Build history of the part. All positions in model axes, mm. Face numbers are marked on the shaded views. A direction names the side the tool comes from. Give positions to 0.01 mm unless a question says otherwise; leave off trailing zeros. Write each loop counter-clockwise with the first axis right and the second up, starting at its lowest first coordinate (ties: lowest second). Pieces come first, ordered by that corner, then holes. Notation, with made-up numbers: (32.5, -9) -> (39.5, -9) arc R16 cw to (39.5, 14) -> close; hole circle Ø8 at (-39, 61). An arc over 180 degrees is marked (long way). Put each result on its own line as item: value.
Autodesk Inventor part; units mm, degrees
ref_plane "YZ Plane" through (0, 0, 0) normal (1, 0, 0) x (0, 1, 0)
ref_plane "XZ Plane" through (0, 0, 0) normal (0, 1, 0) x (-1, 0, 0)
ref_plane "XY Plane" through (0, 0, 0) normal (0, 0, 1) x (1, 0, 0)
sketch "Sketch1" plane through (0, 0, 0) normal (0, 0, 1) x (1, 0, 0)
  line L0 (-3.525, -2.075) -> (3.525, -2.075)
  line L1 (3.525, -2.075) -> (3.525, 2.075)
  line L2 (3.525, 2.075) -> (-3.525, 2.075)
  line L3 (-3.525, 2.075) -> (-3.525, -2.075)
  line L4 (-3.525, -2.075) -> (3.525, 2.075) construction
  line L5 (3.525, -2.075) -> (-3.525, 2.075) construction
  line L6 (-2.925, -1.1225) -> (2.405, -1.1225)
  line L7 (2.405, -1.1225) -> (2.405, 0.1475)
  line L8 (2.405, 0.1475) -> (-2.925, 0.1475)
  line L9 (-2.925, 0.1475) -> (-2.925, -1.1225)
  point P0 (0, 0)
  dimension "d0" = 4.15
  dimension "d1" = 7.05
  dimension "d2" = 5.33
  dimension "d3" = 0.6
  dimension "d4" = 1.27
  dimension "d5" = 0.9525
extrude "Extrusion1" add sketch "Sketch1" along normal mid plane 1.5
sketch "Sketch2" plane through (-3.525, -2.075, 0.75) normal (0, -1, 0) x (1, 0, 0)
  line L0 (7.05, 0.3891) -> (7.05, -1.8891)
  line L1 (7.05, -1.8891) -> (5.4391, -3.5)
  line L2 (5.4391, -3.5) -> (3.1609, -3.5)
  line L3 (3.1609, -3.5) -> (1.55, -1.8891)
  line L4 (1.55, -1.8891) -> (1.55, 0.3891)
  line L5 (1.55, 0.3891) -> (3.1609, 2)
  line L6 (3.1609, 2) -> (5.4391, 2)
  line L7 (5.4391, 2) -> (7.05, 0.3891)
  line L8 (7.05, -1.5) -> (7.05, 0)
  line L9 (3.825, -0.33) -> (3.825, 0.1)
  line L10 (3.825, 0.1) -> (4.775, 0.1)
  line L11 (4.775, 0.1) -> (4.775, -0.33)
  line L12 (4.775, -0.33) -> (6.275, -0.33)
  line L13 (6.275, -0.33) -> (6.275, -1.17)
  line L14 (6.275, -1.17) -> (4.775, -1.17)
  line L15 (4.775, -1.17) -> (4.775, -1.6)
  line L16 (4.775, -1.6) -> (3.825, -1.6)
  line L17 (3.825, -1.6) -> (3.825, -1.17)
  line L18 (3.825, -1.17) -> (2.325, -1.17)
  line L19 (2.325, -1.17) -> (2.325, -0.33)
  line L20 (2.325, -0.33) -> (3.825, -0.33)
  line L21 (4.3, 0.1) -> (4.3, -1.6) construction
  line L22 (2.325, -0.75) -> (6.275, -0.75) construction
  point P0 (3.525, -0.75)
  point P1 (4.3, -0.75)
  dimension "d8" = 5.5
  dimension "d9" = 3.95
  dimension "d10" = 1.7
  dimension "d11" = 0.84
  dimension "d12" = 0.95
extrude "Extrusion2" add sketch "Sketch2" against normal blind 0.65 contours L0 L1 L2 L3 L4 L5 L6 L7 | L9 L10 L11 L12 L13 L14 L15 L16 L17 L18 L19 L20
extrude "Extrusion3" add sketch "Sketch2" along normal blind 3.3 contours L9 L10 L11 L12 L13 L14 L15 L16 L17 L18 L19 L20
properties part number "Replacement latch"
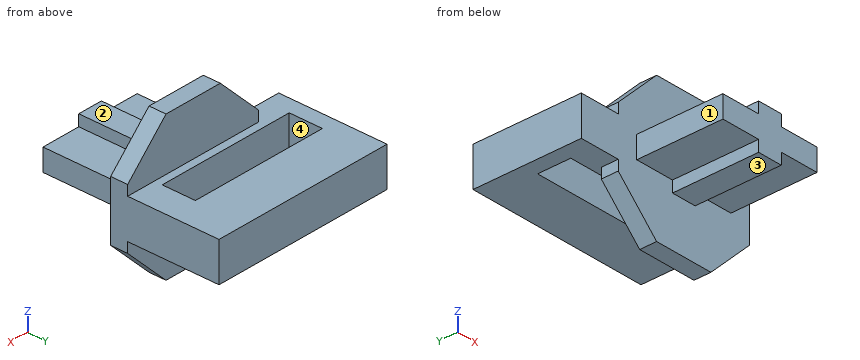
1) Wall check: L1, parallel to Y at x = -2.5, z = -0.05 (1 decimal); L2, parallel to Y at x = 0, z = -0.15 (1 decimal); L3, parallel to Y at x = 1.75, z = 1.35 (3 decimals). Give the ranges that are in metal, low to high.
Filled sheet:
L1: -2.1 to -1.1, 0.1 to 2.1
L2: -5.4 to -1.1, 0.1 to 2.1
L3: -2.075 to -1.425
2) Tool access for the marked faces 1, 2, 3 and 4: list every direction of +Z, -Z, +X, -X, +Y, -Y with a clear straight run to the whole face (end or side of a thin tool).
Filled sheet:
face 1: +Z, -Z, -X, -Y
face 2: +Z, +X, -X, -Y
face 3: -Z, +X, -X, -Y
face 4: +Z, -Z
3) Slice it at D-D (y = -2.75). Write the cut outline in (x, z), plus the area to 4 significant figures.
Filled sheet:
outline: (-1.2, -0.42) -> (0.3, -0.42) -> (0.3, -0.85) -> (1.25, -0.85) -> (1.25, -0.42) -> (2.75, -0.42) -> (2.75, 0.42) -> (1.25, 0.42) -> (1.25, 0.85) -> (0.3, 0.85) -> (0.3, 0.42) -> (-1.2, 0.42) -> close
area: 4.135 mm2
4) Pin check, flat tips, straight feed: pin 1 (1 mm diameter, centred on x = -1, z = 2, fed in from +Y) (3 decimals); pin 2 (0.9 mm diameter, centred on y = -3.5, z = 0, fed in from +X); pin 3 (1 mm diameter, centred on x = 1, y = -3, fed in from +Z). Stop position of each tip, or through.
Filled sheet:
pin 1: y = -1.425
pin 2: x = 2.75
pin 3: z = 0.85
5) Slice it at B-B (y = -0.25). Write the cut outline in (x, z) (3 decimals).
Filled sheet:
outline: (-3.525, -0.75) -> (-2.925, -0.75) -> (-2.925, 0.75) -> (-3.525, 0.75) -> close; (2.405, -0.75) -> (3.525, -0.75) -> (3.525, 0.75) -> (2.405, 0.75) -> close
